Check sheet for the modelled part. Datum: model origin and axes. Units: mm. A direction names the side the tool comes from. Round coordinates to 2 decimals unless told otherwise and drop trailing zeros. Loops run counter-clockwise (first coordinate to the right, second up) from the corner with the lowest first, then second, coordinate; pieces in that order, holes last. Notation, with made-up numbers: (-2, 18) -> (13, 18) arc R25 cw to (13, 38) -> close; hole circle Ø9 at (84.5, 12). An arc over 180 degrees is marked (long way). Return JSON: item names as keys, results as strings.
Autodesk Inventor part; units mm, degrees
ref_plane "YZ Plane" through (0, 0, 0) normal (1, 0, 0) x (0, 1, 0)
ref_plane "XZ Plane" through (0, 0, 0) normal (0, 1, 0) x (-1, 0, 0)
ref_plane "XY Plane" through (0, 0, 0) normal (0, 0, 1) x (1, 0, 0)
sketch "Sketch1" plane through (0, 0, 0) normal (0, 0, 1) x (1, 0, 0)
  line L0 (28.8, -21.6) -> (-28.8, -21.6)
  line L1 (-28.8, -21.6) -> (-28.8, 21.6)
  line L2 (-28.8, 21.6) -> (28.8, 21.6)
  line L3 (28.8, 21.6) -> (28.8, -21.6)
  line L4 (28.8, -21.6) -> (-28.8, 21.6) construction
  line L5 (-28.8, -21.6) -> (28.8, 21.6) construction
  line L6 (-34.3, -26.7) -> (34.3, -26.7)
  line L7 (34.3, -26.7) -> (34.3, 26.7)
  line L8 (34.3, 26.7) -> (-34.3, 26.7)
  line L9 (-34.3, 26.7) -> (-34.3, -26.7)
  line L10 (-34.3, -26.7) -> (34.3, 26.7) construction
  line L11 (34.3, -26.7) -> (-34.3, 26.7) construction
  line L12 (-40.65, 33.05) -> (40.65, 33.05)
  line L13 (40.65, 33.05) -> (40.65, -33.05)
  line L14 (40.65, -33.05) -> (-40.65, -33.05)
  line L15 (-40.65, -33.05) -> (-40.65, 33.05)
  line L16 (-50.8, -33.05) -> (50.8, -33.05)
  line L17 (50.8, -33.05) -> (50.8, 33.05)
  line L18 (50.8, 33.05) -> (-50.8, 33.05)
  line L19 (-50.8, 33.05) -> (-50.8, -33.05)
  line L20 (-50.8, -33.05) -> (50.8, 33.05) construction
  line L21 (50.8, -33.05) -> (-50.8, 33.05) construction
  point P0 (0, 0)
  dimension "d0" = 43.2
  dimension "d1" = 57.6
  dimension "d2" = 68.6
  dimension "d3" = 53.4
  dimension "d4" = 6.35
  dimension "d7" = 101.6
  dimension "d8" = 66.1
extrude "Extrusion1" add sketch "Sketch1" along normal blind 17.4625 contours L9 L8 L7 L6 | L12 L13 L14 L15 | L15 L16 L19 L18 | L18 L17 L16 L13
shell "Shell1" thickness 1 removed faces 5 at (-43.4667, 7.2, 17.4625) at (-28.8, -7.2, 5.8208) at (-9.6, 21.6, 5.8208) at (28.8, 7.2, 5.8208) at (9.6, -21.6, 5.8208)
fillet "Fillet1" radius 12.7 2 edges at (-50.8, 0, 0) (50.8, 0, 0)
sketch "Sketch2" plane through (-50.8, 33.05, 17.4625) normal (0, 1, 0) x (1, 0, 0)
  arc A0 (101.6, 4.7625) -> (88.9, 17.4625) centre (88.9, 4.7625) ccw
  line L0 (88.9, 17.4625) -> (12.7, 17.4625)
  arc A1 (12.7, 17.4625) -> (0, 4.7625) centre (12.7, 4.7625) ccw
  line L1 (0, 4.7625) -> (0, 0)
  line L2 (101.6, 0) -> (0, 0)
  line L3 (101.6, 4.7625) -> (101.6, 0)
  line L4 (101.6, 0) -> (0, 0) construction
  line L5 (50.8, 0) -> (50.8, 17.4625) construction
  line L6 (57.15, 17.4625) -> (44.45, 17.4625)
  line L7 (44.45, 17.4625) -> (44.45, 0)
  line L8 (44.45, 0) -> (57.15, 0)
  line L9 (57.15, 0) -> (57.15, 17.4625)
  dimension "d11" = 12.7
extrude "Extrusion2" add sketch "Sketch2" along normal blind 12.7 contours L9 L2 L7 L0
sketch "Sketch3" plane through (0, 0, 0) normal (0, 0, -1) x (-1, 0, 0)
  line L0 (-38.1, -33.05) -> (-38.1, 33.05)
  line L1 (38.1, -33.05) -> (-38.1, -33.05)
  line L2 (38.1, 33.05) -> (38.1, -33.05)
  line L3 (6.35, 33.05) -> (38.1, 33.05)
  line L4 (6.35, 33.05) -> (6.35, 45.75)
  line L5 (-6.35, 45.75) -> (6.35, 45.75)
  line L6 (-6.35, 33.05) -> (-6.35, 45.75)
  line L7 (-38.1, 33.05) -> (-6.35, 33.05)
  line L8 (28.8, 21.6) -> (28.8, -21.6)
  line L9 (28.8, -21.6) -> (-28.8, -21.6)
  line L10 (-28.8, -21.6) -> (-28.8, 21.6)
  line L11 (-28.8, 21.6) -> (28.8, 21.6)
  line L12 (-6.35, 45.75) -> (6.35, 33.05) construction
  line L13 (6.35, 33.05) -> (6.35, 45.75) construction
  line L14 (6.35, 45.75) -> (-6.35, 33.05) construction
  point P0 (0, 0)
  point P1 (0, 39.4)
hole "Hole1" at (0, 39.4, 0) direction (0, 0, 1) diameter 9.525 end through all
fillet "Fillet2" radius 12.7 2 edges at (-49.8, 0, 1) (49.8, 0, 1)
equation "\"d8\" = 2 * d4 + d3"
properties part number "Back"
Q1. Go/stop test with flat-tipped pins: pin 1 (6.5 mm diameter, centred on y = 39, z = 5.5, fed in from -X); pin 2 (10 mm diameter, centred on x = -6.5, z = 13.5, fed in from +Y); pin 3 (8.5 mm diameter, centred on x = -17.5, z = 10.5, fed in from +Y); pin 4 (2 mm diameter, centred on y = 15.5, z = 10, fed in from +X). Record where each tip stops, or that it passes through.
Results list:
{"pin 1": "x = -6.35", "pin 2": "y = 45.75", "pin 3": "y = 33.05", "pin 4": "x = 50.69"}
Q2. Section check D-D (x = 26.5). Record the boundary of the cut face in (y, z), then the cut area to 3 significant figures.
Results list:
{"outline": "(-33.05, 0) -> (-21.6, 0) -> (-21.6, 1) -> (-32.05, 1) -> (-32.05, 17.46) -> (-33.05, 17.46) -> close; (21.6, 0) -> (33.05, 0) -> (33.05, 17.46) -> (32.05, 17.46) -> (32.05, 1) -> (21.6, 1) -> close", "area": "55.8 mm^2"}
Q3. Draft check along Y on faces 1 (the flat face through (0, 45.75, 9)), 2 (the flat face through (6.35, 39, 9)), 3 (the cylindrical face through (-45.98, 0.45, 4.62)). Enter one of: released by +Y, released by -Y, zero draft, split by the parting line, or undercut.
Results list:
{"face 1": "released by +Y", "face 2": "zero draft", "face 3": "undercut"}
Q4. Section check B-B (y = 9). Record the boundary of the cut face in (x, z), then the cut area to 3 significant figures.
Results list:
{"outline": "(-50.8, 12.7) arc R12.7 ccw to (-38.1, 0) -> (-28.8, 0) -> (-28.8, 1) -> (-37.1, 1) arc R12.7 cw to (-49.8, 13.7) -> (-49.8, 17.46) -> (-50.8, 17.46) -> close; (28.8, 0) -> (38.1, 0) arc R12.7 ccw to (50.8, 12.7) -> (50.8, 17.46) -> (49.8, 17.46) -> (49.8, 13.7) arc R12.7 cw to (37.1, 1) -> (28.8, 1) -> close", "area": "76.9 mm^2"}
Q5. Section check A-A (x = 0). Record the boundary of the cut face in (y, z), then the cut area to 3 significant figures.
Results list:
{"outline": "(-33.05, 0) -> (-21.6, 0) -> (-21.6, 1) -> (-32.05, 1) -> (-32.05, 17.46) -> (-33.05, 17.46) -> close; (21.6, 0) -> (34.64, 0) -> (34.64, 17.46) -> (32.05, 17.46) -> (32.05, 1) -> (21.6, 1) -> close; (44.16, 0) -> (45.75, 0) -> (45.75, 17.46) -> (44.16, 17.46) -> close", "area": "111 mm^2"}
Q6. Tool access check on faces 4 (the cylindrical face through (45.98, -0.45, 4.62)), 5 (the flat face through (0, 33, 17.462)), 6 (the flat face through (-6.35, 39, 9)). Record the directions out of +Z, -Z, +X, -X, +Y, -Y that give a thin tool (end or side, any length) a straight path to the whole face; none if there is none.
Results list:
{"face 4": "+Z", "face 5": "+Z, +X, -X, +Y, -Y", "face 6": "+Z, -Z, -X, +Y"}
Q7. Material ranges on line 1 (Y direction, x = 0, z = 8); line 2 (Y direction, x = -16.5, z = 11.75); line 3 (X direction, y = 39.5, z = 12.5), recorded low to high.
Results list:
{"line 1": "-33.05 to -32.05, 32.05 to 34.64, 44.16 to 45.75", "line 2": "-33.05 to -32.05, 32.05 to 33.05", "line 3": "-6.35 to -4.76, 4.76 to 6.35"}
Q8. Section check C-C (z = 5). Count the separate pieces of the cut face and the enclosed holes in it, then the cut area to 3 significant figures.
Results list:
{"separate pieces": "1", "enclosed holes": "2", "area": "520 mm^2"}
